Read the model definition and answer for the solid it produces. Units are mm, in the model's axes. Face numbers are marked on the shaded views. Give positions to 0.01 mm unless a question says otherwise; leave off trailing zeros. Order: outer loops, then holes, each group sorted by start corner. A loop starts at its lowest first (then second) coordinate and runs counter-clockwise, first axis right, second up.
Item 1: A cutting plane is placed at A-A (z = 10.25). Write down the section's boundary in (x, y).
Item 2: Find the intervals of material crossed by line 1 along X through (y, z) = (-88, 10.25); line 2 along X through (y, z) = (-88, 3.25); line 3 along X through (y, z) = (-85, 2.75), in increasing order.
Item 3: Given pin 1 Ø0.6 at (x, z) = (64.5, 1) entering from +Y; pin 2 Ø0.6 at (x, z) = (80, 0.5) entering from -Y; pin 3 Ø4 at (x, y) = (64.18, -88.03) entering from -Z, each flat-ended and moving along its own axis, determine where each tip first touches the part or whether it passes through.
Item 4: The mould has two halves that part along X. Classify the marked faces 1, 2 and 3: +X half, -X half, draft (parallel to the pull), parting line (faces both ways), or undercut.
Item 5: A cutting plane is placed at C-C (x = 117). Write down the section's boundary in (y, z), plus the area to 4 significant figures.
Item 6: A cutting plane is placed at B-B (y = -97). Write down the section's boundary in (x, z), plus the area to 3 significant figures.
from build123d import *

# Parameters (mm, degrees)
CROQUIS1_W                      = 140
CROQUIS1_H                      = 37.125
CROQUIS1_R                      = 1.625
SALIENTE_EXTRUIR1_DEPTH         = 4
CROQUIS2_R                      = 3.35997123
CORTAR_EXTRUIR1_DEPTH           = 1.8
CORTAR_EXTRUIR1_DRAFT           = -44
CORTAR_EXTRUIR1_PROFILE_2_DEPTH = 1.8
CORTAR_EXTRUIR1_PROFILE_2_DRAFT = -44
CROQUIS3_R                      = 1.625
CORTAR_EXTRUIR2_DEPTH           = 4
SALIENTE_EXTRUIR2_DEPTH         = 10
CROQUIS6_W                      = 13.9
CROQUIS6_H                      = 11.4
SALIENTE_EXTRUIR4_DEPTH         = 2
CORTAR_EXTRUIR3_DEPTH           = 2
CORTAR_EXTRUIR4_START           = -140
CORTAR_EXTRUIR4_DEPTH           = 140


with BuildPart() as part:
    # Croquis1 → Saliente-Extruir1 (new body)
    with BuildSketch(Plane.XY):
        with Locations((62.679008317, -85.846623552)):
            Rectangle(CROQUIS1_W, CROQUIS1_H)
        with Locations((122.679008317, -87.284123552)):
            Circle(CROQUIS1_R, mode=Mode.SUBTRACT)
        with Locations((2.679008317, -87.284123552)):
            Circle(CROQUIS1_R, mode=Mode.SUBTRACT)
    extrude(amount=SALIENTE_EXTRUIR1_DEPTH)


with BuildPart() as cortar_extruir1_tool:
    # Croquis2 → Cortar-Extruir1 (with draft: the straight prism first)
    with BuildSketch(Plane.XY.offset(4)):
        with Locations((2.679008317, -87.284123552)):
            Circle(CROQUIS2_R)
    extrude(amount=-CORTAR_EXTRUIR1_DEPTH)
    # Cortar-Extruir1: the draft: its side faces are tilted about the plane it starts from
    cortar_extruir1_sides = [cortar_extruir1_tool.faces().sort_by_distance(p)[0] for p in [
        (-0.680962913, -87.284123552, 3.1),
    ]]
    draft(cortar_extruir1_sides, Plane.XY.offset(4), CORTAR_EXTRUIR1_DRAFT)


with BuildPart() as part_1:
    add(part.part)

    # Cortar-Extruir1: cut by cortar_extruir1_tool
    add(cortar_extruir1_tool.part, mode=Mode.SUBTRACT)


with BuildPart() as cortar_extruir1_profile_2_tool:
    # Croquis2 → Cortar-Extruir1 profile 2 (with draft: the straight prism first)
    with BuildSketch(Plane.XY.offset(4)):
        with Locations((122.679008317, -87.284123552)):
            Circle(CROQUIS2_R)
    extrude(amount=-CORTAR_EXTRUIR1_PROFILE_2_DEPTH)
    # Cortar-Extruir1 profile 2: the draft: its side faces are tilted about the plane it starts from
    cortar_extruir1_profile_2_sides = [cortar_extruir1_profile_2_tool.faces().sort_by_distance(p)[0] for p in [
        (119.319037087, -87.284123552, 3.1),
    ]]
    draft(cortar_extruir1_profile_2_sides, Plane.XY.offset(4), CORTAR_EXTRUIR1_PROFILE_2_DRAFT)


with BuildPart() as part_2:
    add(part_1.part)

    # Cortar-Extruir1 profile 2: cut by cortar_extruir1_profile_2_tool
    add(cortar_extruir1_profile_2_tool.part, mode=Mode.SUBTRACT)

    # Croquis3 → Cortar-Extruir2 (cut)
    with BuildSketch(Plane.XY.offset(4)):
        with Locations((80.609008317, -84.449123552)):
            Circle(CROQUIS3_R)
        with Locations((108.469008317, -84.454123552)):
            Circle(CROQUIS3_R)
        with Locations((34.179008317, -72.034123552)):
            Circle(CROQUIS3_R)
        with Locations((64.179008317, -88.034123552)):
            Circle(CROQUIS3_R)
    extrude(amount=-CORTAR_EXTRUIR2_DEPTH, mode=Mode.SUBTRACT)

    # Croquis4 → Saliente-Extruir2 (add)
    with BuildSketch(Plane.XY.offset(4)):
        Polygon((13.170968426, -85.674315594), (13.170968426, -88.674315594), (7.179008317, -88.674315594), (7.179008317, -74.274315594), (9.179008317, -74.274315594), (9.179008317, -85.674315594), align=None)
        Polygon((19.129008317, -85.674315594), (19.138778044, -88.674315594), (25.079008317, -88.674315594), (25.079008317, -74.274315594), (23.079008317, -74.274315594), (23.079008317, -85.674315594), align=None)
    extrude(amount=SALIENTE_EXTRUIR2_DEPTH)

    # Croquis6 → Saliente-Extruir4 (add)
    with BuildSketch(Plane.XY.offset(4)):
        with Locations((16.129008317, -79.974315594)):
            Rectangle(CROQUIS6_W, CROQUIS6_H)
    extrude(amount=SALIENTE_EXTRUIR4_DEPTH)

    # Croquis8 → Cortar-Extruir3 (cut)
    with BuildSketch(Plane(origin=(0, 0, 0), x_dir=(-1, 0, 0), z_dir=(0, 0, -1))):
        Polygon((-105.299008317, -84.454123552), (-106.884008317, -81.708823022), (-110.054008317, -81.708823022), (-111.639008317, -84.454123552), (-110.054008317, -87.199424082), (-106.884008317, -87.199424082), align=None)
        Polygon((-61.009008317, -88.034123552), (-62.594008317, -85.288823022), (-65.764008317, -85.288823022), (-67.349008317, -88.034123552), (-65.764008317, -90.779424082), (-62.594008317, -90.779424082), align=None)
        Polygon((-77.439008317, -84.449123552), (-79.024008317, -81.703823022), (-82.194008317, -81.703823022), (-83.779008317, -84.449123552), (-82.194008317, -87.194424082), (-79.024008317, -87.194424082), align=None)
        Polygon((-31.009008317, -72.034123552), (-32.594008317, -69.288823022), (-35.764008317, -69.288823022), (-37.349008317, -72.034123552), (-35.764008317, -74.779424082), (-32.594008317, -74.779424082), align=None)
    extrude(amount=-CORTAR_EXTRUIR3_DEPTH, mode=Mode.SUBTRACT)

    # Croquis9 → Cortar-Extruir4 (cut)
    with BuildSketch(Plane.ZY.offset(7.320991683).offset(CORTAR_EXTRUIR4_START)):
        Polygon((4, -104.409123552), (0, -104.409123552), (4, -100.409123552), align=None)
        Polygon((0, -67.284123552), (4, -67.284123552), (4, -69.284123552), align=None)
    extrude(amount=CORTAR_EXTRUIR4_DEPTH, mode=Mode.SUBTRACT)


solid = part_2.part
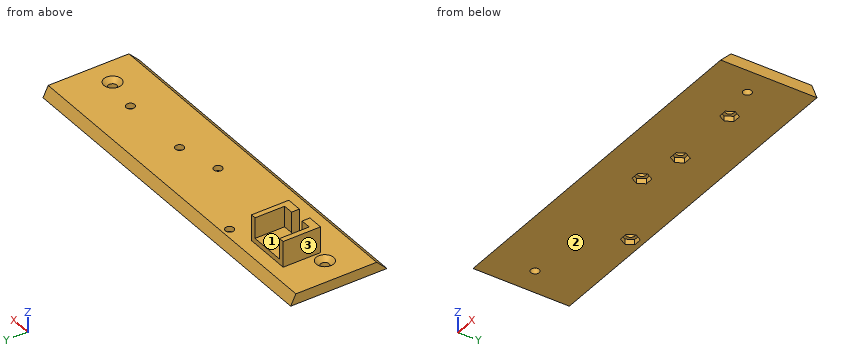
Response values:
1. outline: (7.18, -88.67) - (13.17, -88.67) - (13.17, -85.67) - (9.18, -85.67) - (9.18, -74.27) - (7.18, -74.27) - close; (19.13, -85.67) - (19.14, -88.67) - (25.08, -88.67) - (25.08, -74.27) - (23.08, -74.27) - (23.08, -85.67) - close
2. line 1: x = 7.18 to 13.17, 19.14 to 25.08
2. line 2: x = -7.32 to 0.14, 5.22 to 62.55, 65.8 to 120.14, 125.22 to 132.68
2. line 3: x = -7.32 to 79.08, 82.14 to 106.94, 110 to 132.68
3. pin 1: stops at y = -67.63
3. pin 2: stops at y = -104.21
3. pin 3: stops at z = 2
4. face 1: undercut
4. face 2: draft
4. face 3: -X half
5. outline: (-104.41, 0) - (-67.28, 0) - (-69.28, 4) - (-100.41, 4) - close
5. area: 136.5 mm2
6. outline: (-7.32, 0) - (132.68, 0) - (132.68, 4) - (-7.32, 4) - close
6. area: 560 mm2
